Here's how the part is built. I have some questions about the finished solid (model axes, mm). A direction names the side the tool comes from. Coordinates: 2 decimals unless noted, no trailing zeros. Write each loop counter-clockwise with the first axis right and the second up, starting at its lowest first coordinate (ties: lowest second). Pieces come first, ordered by that corner, then holes. Notation, with made-up numbers: (37, -19) -> (93, -19) arc R27 ccw to (93, 11) -> close; hole circle Ø5 at (-18.75, 83). An arc over 180 degrees is marked (long way). Put each result on its own line as item: value. Start each with the question number.
Item 1: I want a section at A-A, the plane y = 0. List the corners of the cut face in (x, z) for me.
Item 2: I want a section at D-D, the plane y = -6.25. List the corners of the cut face in (x, z) for me, then the cut area to 3 significant figures.
Item 3: I need wall thicknesses on line 1 (Y direction, x = 0, z = 1.5); line 2 (X direction, y = 0.75, z = 0.75); line 3 (Y direction, x = -1, z = 1.5). Which ranges of each line are inside material? Lowest first, please. Write a range as [from, to].
Item 4: I want a section at C-C, the plane z = 6.25. List the corners of the cut face in (x, y) for me.
Item 5: For pin 1 (2.5 mm diameter, centred on x = 1.81, y = 6.76, fed in from -Z); pin 2 (1 mm diameter, centred on x = 4.5, z = 5.5, fed in from -Y); pin 3 (1 mm diameter, centred on x = 4.95, y = -4.95, fed in from +Z); pin 4 (2 mm diameter, centred on x = 4, z = 4, fed in from +Y), each with a flat end and sliding along its axis, tell me the tip position at first contact or that it passes through.
Item 6: I want a section at B-B, the plane x = 0. List the corners of the cut face in (y, z) for me.
Item 7: On a 3-axis mill with a long thin cutter (end or side, diameter ignored), from which of +Z, -Z, +X, -X, +Y, -Y can I reach the whole of each face in a straight line? I mean faces 1 (the face through (-2.87, 2.64, 0.3)), 2 (the face through (0, 0, 6.5)). Say none if no direction works.
Item 8: If we mould it in two halves opening along X, with no side actions, what happens to faces 3 (the face through (-4, -6, 0)), 4 (the face through (-2.17, -9.76, 3.2)), 5 (the face through (1.57, 6, 4.01))? For each: released by +X, released by -X, zero draft, split by the parting line, or undercut.
from build123d import *

# Parameters (mm, degrees)
CYLINDER044_R            = 0.8
CYLINDER044_DEPTH        = 10
ARRAY007_COUNT           = 3
ARRAY007_PLACEMENT_ANGLE = 45
CYLINDER027_R            = 4.55
CYLINDER027_DEPTH        = 10
CYLINDER026_R            = 3.9
CYLINDER026_DEPTH        = 10
CYLINDER024_R            = 1.4
CYLINDER024_DEPTH        = 10
ARRAY_COUNT              = 3
CYLINDER023_R            = 9
CYLINDER023_DEPTH        = 1.59
CYLINDER043_R            = 10
CYLINDER043_DEPTH        = 6.5


with BuildPart() as array007:
    # Cylinder044 → Cylinder044 (new body)
    with BuildSketch(Plane(origin=(7, 0, 0), x_dir=(1, 0, 0), z_dir=(0, 0, 1))):
        Circle(CYLINDER044_R)
    extrude(amount=CYLINDER044_DEPTH)

    # Array007: Array007 ×3 about axis
    array007_axis = Axis((0, 0, 0), (0, 0, 1))


with BuildPart() as array007_1:
    add(array007.part)
    for i in range(1, ARRAY007_COUNT):
        add(array007.part.rotate(array007_axis, i * 360 / ARRAY007_COUNT))


with BuildPart() as array007_2:
    # Array007 placement: moved
    add(array007_1.part.rotate(Axis((0, 0, 0), (0, 0, -1)), ARRAY007_PLACEMENT_ANGLE))


with BuildPart() as mountplatelip:
    # Cylinder027 → Cylinder027 (new body)
    with BuildSketch(Plane.XY.offset(0.6)):
        Circle(CYLINDER027_R)
    extrude(amount=CYLINDER027_DEPTH)


with BuildPart() as mountplateinnerhole:
    # Cylinder026 → Cylinder026 (new body)
    with BuildSketch(Plane.XY):
        Circle(CYLINDER026_R)
    extrude(amount=CYLINDER026_DEPTH)


with BuildPart() as fusion012:
    # Cylinder024 → Cylinder024 (new body)
    with BuildSketch(Plane(origin=(8, 0, 0), x_dir=(1, 0, 0), z_dir=(0, 0, 1))):
        Circle(CYLINDER024_R)
    extrude(amount=CYLINDER024_DEPTH)

    # Array: Fusion012 ×3 about axis
    array_axis = Axis((0, 0, 0), (0, 0, 1))


with BuildPart() as fusion012_1:
    add(fusion012.part)
    for i in range(1, ARRAY_COUNT):
        add(fusion012.part.rotate(array_axis, i * 360 / ARRAY_COUNT))

    # Fusion012: union MountPlateLip, MountPlateInnerHole
    add(mountplatelip.part)
    add(mountplateinnerhole.part)


with BuildPart() as cut013:
    # Cylinder023 → Cylinder023 (new body)
    with BuildSketch(Plane.XY):
        Circle(CYLINDER023_R)
    extrude(amount=CYLINDER023_DEPTH)

    # Cut013: cut Fusion012
    add(fusion012_1.part, mode=Mode.SUBTRACT)


with BuildPart() as cut015:
    # Cylinder043 → Cylinder043 (new body)
    with BuildSketch(Plane.XY):
        Circle(CYLINDER043_R)
    extrude(amount=CYLINDER043_DEPTH)

    # Cut014: cut Cut013
    add(cut013.part, mode=Mode.SUBTRACT)

    # Cut015: cut Array007
    add(array007_2.part, mode=Mode.SUBTRACT)


solid = cut015.part
Calculated:
1. outline: (-10, 0) -> (-9, 0) -> (-9, 1.59) -> (-4.55, 1.59) -> (-4.55, 0.6) -> (-3.9, 0.6) -> (-3.9, 0) -> (3.9, 0) -> (3.9, 0.6) -> (4.55, 0.6) -> (4.55, 1.59) -> (6.6, 1.59) -> (6.6, 0) -> (10, 0) -> (10, 6.5) -> (-10, 6.5) -> close
2. outline: (-7.81, 0) -> (-6.48, 0) -> (-6.48, 1.59) -> (-5.22, 1.59) -> (-5.22, 0) -> (-2.78, 0) -> (-2.78, 1.59) -> (6.48, 1.59) -> (6.48, 0) -> (7.81, 0) -> (7.81, 6.5) -> (-7.81, 6.5) -> close
2. area: 84.8 mm2
3. line 1: y = [-10, -9], [-4.55, 4.55], [9, 10]
3. line 2: x = [-9.97, -8.97], [-4.49, 4.49], [6.82, 9.97]
3. line 3: y = [-9.95, -8.94], [-4.44, 4.44], [8.94, 9.95]
4. outline: circle Ø20 at (0, 0); hole circle Ø1.6 at (-6.76, -1.81); hole circle Ø1.6 at (1.81, 6.76); hole circle Ø1.6 at (4.95, -4.95)
5. pin 1: stops at z = 1.59
5. pin 2: stops at y = -9.17
5. pin 3: passes through
5. pin 4: stops at y = 9.54
6. outline: (-10, 0) -> (-9, 0) -> (-9, 1.59) -> (-4.55, 1.59) -> (-4.55, 0.6) -> (-3.9, 0.6) -> (-3.9, 0) -> (3.9, 0) -> (3.9, 0.6) -> (4.55, 0.6) -> (4.55, 1.59) -> (9, 1.59) -> (9, 0) -> (10, 0) -> (10, 6.5) -> (-10, 6.5) -> close
7. face 1: -Z
7. face 2: +Z, +X, -X, +Y, -Y
8. face 3: zero draft
8. face 4: split by the parting line
8. face 5: undercut
